Part model, mm, in its own coordinate system. Face numbers are marked on the shaded views. A direction names the side the tool comes from. Round coordinates to 2 decimals unless told otherwise and drop trailing zeros. Loops run counter-clockwise (first coordinate to the right, second up) from the corner with the lowest first, then second, coordinate; pieces in that order, holes last. Notation, with made-up numbers: (69, -40) -> (79, -40) arc R31 cw to (79, -10) -> close; hole circle Ø8 at (89.25, -7.5). An arc over 180 degrees is marked (long way). Answer as a JSON object with one key per item and string values. Group by question number.
from build123d import *

# Parameters (mm, degrees)
EXTRUDE_1_DEPTH       = 8
SKETCH_2_W            = 3.75
SKETCH_2_H            = 1.5
CUT_EXTRUDE_1_DEPTH   = 13.896220377
SKETCH_3_W            = 3.75
SKETCH_3_H            = 1.5
CUT_EXTRUDE_2_DEPTH   = 13.896220377
HOLE_WIZARD_6_0_6_1_D = 6
CHAMFER_1_SIZE        = 0.5
FILLET_1_R            = 1
FILLET_2_R            = 2
FILLET_3_R            = 3
FILLET_4_R            = 4


with BuildPart() as part:
    # 草图1 → 凸台-拉伸1 (new body)
    with BuildSketch(Plane(origin=(0, 4, 0), x_dir=(1, 0, 0), z_dir=(0, 1, 0))):
        Polygon((-7.75, -3), (-7.75, -6.5), (7.75, -6.5), (7.75, -3), (4.75, 0), (-4.75, 0), align=None)
    extrude(amount=-EXTRUDE_1_DEPTH)

    # 草图2 → 切除-拉伸1 (cut, through all)
    with BuildSketch(Plane.XZ.offset(4)):
        with Locations((-5.875, 5.75)):
            Rectangle(SKETCH_2_W, SKETCH_2_H)
    extrude(amount=-CUT_EXTRUDE_1_DEPTH, mode=Mode.SUBTRACT)

    # 草图3 → 切除-拉伸2 (cut, through all)
    with BuildSketch(Plane.XZ.offset(4)):
        with Locations((5.875, 5.75)):
            Rectangle(SKETCH_3_W, SKETCH_3_H)
    extrude(amount=-CUT_EXTRUDE_2_DEPTH, mode=Mode.SUBTRACT)

    # Ø6.0 (6) 直径孔1 (through all)
    with Locations(Plane(origin=(0, 0, 0), x_dir=(-1, 0, 0), z_dir=(0, 0, -1))):
        with Locations((0, 0)):
            Hole(HOLE_WIZARD_6_0_6_1_D / 2)

    # 倒角1
    chamfer_1_edges = [part.edges().sort_by_distance(p)[0] for p in [
        (-3, 0, 0),
        (-3, 0, 6.5),
    ]]
    chamfer(chamfer_1_edges, length=CHAMFER_1_SIZE)

    # 圆角1
    fillet_1_edges = [part.edges().sort_by_distance(p)[0] for p in [
        (7.75, 4, 4),
        (-7.75, -4, 4),
    ]]
    fillet(fillet_1_edges, radius=FILLET_1_R)

    # 圆角2
    fillet_2_edges = [part.edges().sort_by_distance(p)[0] for p in [
        (-4.75, 0, 0),
        (4.75, 0, 0),
    ]]
    fillet(fillet_2_edges, radius=FILLET_2_R)

    # 圆角3
    fillet_3_edges = [part.edges().sort_by_distance(p)[0] for p in [
        (7.75, -4, 4),
        (-7.75, 4, 4),
    ]]
    fillet(fillet_3_edges, radius=FILLET_3_R)

    # 圆角4
    fillet_4_edges = [part.edges().sort_by_distance(p)[0] for p in [
        (-4, 4, 5.75),
        (4, -4, 5.75),
    ]]
    fillet(fillet_4_edges, radius=FILLET_4_R)


solid = part.part
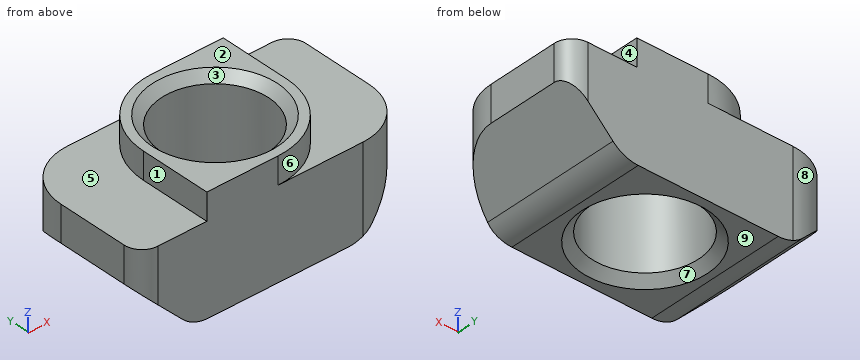
Item 1: Drill centre lines: line 1 (Y direction, x = 0, z = 1.95); line 2 (Y direction, x = -1.5, z = 1.25); line 3 (X direction, y = 2, z = 1). Where is each one in solid material? Low to high.
Item 2: Band-saw the part on D-D, the plane z = 2.25. List the corners of the cut face in (x, y), plus the area to 3 significant figures.
Item 3: Band-saw the part on C-C, the plane x = -5.75. List the corners of the cut face in (y, z), plus the area to 3 significant figures.
Item 4: Drop flat-ended pins along their axis: pin 1 Ø1.5 at (y, z) = (-2, 1) entering from +X; pin 2 Ø1.6 at (y, z) = (2, 6) entering from +X. Give the stop position or say it passes through.
Item 5: Which spindle directions (+Z, -Z, +X, -X, +Y, -Y) get a long thin tool onto all of the face, cutting with end or side? Do the marked faces 1, 2, 3, 4 and 5. Say none if no direction does.
Item 6: Band-saw the part on A-A, the plane z = 6.25. List the corners of the cut face in (x, y).
Item 7: Two-plate mould, pull along X, no slides. Class the marked faces 6, 7, 8 and 9: pulls with the +X half, pulls with the -X half, needs draft (parallel to the pull), parting line crosses it, or undercut.
Item 8: Band-saw the part on B-B, the plane z = 1.5. List the corners of the cut face in (x, y), plus the area to 3 significant figures.
Entries:
{
 "1": {"line 1": "-4 to -3, 3 to 4", "line 2": "-4 to -2.6, 2.6 to 4", "line 3": "-5.75 to -2.24, 2.24 to 5.75"},
 "2": {"outline": "(-7, -3.97) arc R1 ccw to (-6.75, -4) -> (4.75, -4) arc R3 ccw to (7, -2.98) -> (7, 3.97) arc R1 ccw to (6.75, 4) -> (-4.75, 4) arc R3 ccw to (-7, 2.98) -> close; hole circle Ø6 at (0, 0)", "area": "82.3 mm²"},
 "3": {"outline": "(-4, 1) -> (3.83, 1) -> (3.83, 5) -> (-4, 5) -> close", "area": "31.3 mm²"},
 "4": {"pin 1": "x = 6.5", "pin 2": "x = 4"},
 "5": {"face 1": "+Z, -X, +Y, -Y", "face 2": "+Z, +X, -X, +Y, -Y", "face 3": "+Z", "face 4": "+Z, +X, +Y, -Y", "face 5": "+Z, -X, +Y"},
 "6": {"outline": "(-4, -4) -> (0, -4) arc R4 ccw to (4, 0) -> (4, 4) -> (0, 4) arc R4 ccw to (-4, 0) -> close; hole circle Ø6.5 at (0, 0)"},
 "7": {"face 6": "pulls with the +X half", "face 7": "undercut", "face 8": "pulls with the -X half", "face 9": "needs draft"},
 "8": {"outline": "(-6.25, -4) -> (4.75, -4) arc R3 ccw to (6.25, -3.6) -> (6.25, 4) -> (-4.75, 4) arc R3 ccw to (-6.25, 3.6) -> close; hole circle Ø6 at (0, 0)", "area": "71.3 mm²"}
}
